Could you check a few things on this model? Use its own coordinates, in mm. A direction names the side the tool comes from. Coordinates: 2 decimals unless noted, no trailing zeros. Order: outer loops, then holes, each group sorted by start corner. A loop starts at its lowest first (then second) coordinate and runs counter-clockwise, first axis right, second up. Notation, with made-up numbers: (-2, -21) - (3, -21) arc R19 ccw to (3, -2) - close; hole circle Ø2 at (57, 7). An arc over 180 degrees is marked (long way). Answer as CSV lines item,"result". Start each with the question number.
1. I need wall thicknesses on probe 1 along X at (y, z) = (1.45, 24.65) (3 decimals); probe 2 along X at (y, z) = (28, 8.5) (3 decimals); probe 3 along Z at (x, y) = (-21, 22). Which ranges of each line are inside material? Lowest first, please.
2. I want a section at D-D, the plane z = -0.5. List the corners of the cut face in (x, y) for me (3 decimals).
3. Thinking about a two-plate mould opening in X: for faces 1 (the face through (38.82, 0.99, -26.08)), 2 (the face through (-49.775, 17, 0)), 3 (the face through (54, 2, -16)), 4 (the face through (39, 2, -24)), which applies, released by +X, released by -X, zero draft, split by the parting line, or undercut?
4. For pin 1 (5 mm diameter, centred on y = 18, z = -15.5, fed in from +X) (3 decimals); pin 2 (2 mm diameter, centred on y = 24.5, z = 2, fed in from -X) (3 decimals); pin 3 (1.3 mm diameter, centred on x = 40, z = -24.5, fed in from -Y), each with a flat end and sliding along its axis, tell me the tip position at first contact or that it passes through.
5. I want a section at C-C, the plane z = 24.65. List the corners of the cut face in (x, y) for me (3 decimals).
6. I want a section at A-A, the plane x = -42. List the corners of the cut face in (y, z) for me, and give its area (3 significant figures).
7. For faces 5 (the face through (50.775, 1, 0)), 6 (the face through (44.761, 0.986, 25.756)), 7 (the face through (53, 10, -16)), which set-ups out of +Z, -Z, +X, -X, +Y, -Y let a thin tool reach every point of the face, with its end or its side?
8. I want a section at B-B, the plane y = 18. List the corners of the cut face in (x, z) for me (3 decimals), and give its area (3 significant figures).
from build123d import *

# Parameters (mm, degrees)
ESBO_O1_W                  = 101.55
ESBO_O1_H                  = 53.3
RESSALTO_EXTRUS_O1_DEPTH   = 2
ESBO_O2_W                  = 53.2
ESBO_O2_H                  = 53.3
RESSALTO_EXTRUS_O2_DEPTH   = 26.416687688
CORTE_EXTRUS_O2_DEPTH      = 64.136079332
CORTE_EXTRUS_O2_DEPTH_BACK = 64.64
ESBO_O5_R                  = 1.5
ESBO_O6_W                  = 99.55
ESBO_O6_H                  = 51.3
RESSALTO_EXTRUS_O4_DEPTH   = 30
ESBO_O7_W                  = 16.925657076
ESBO_O7_H                  = 8.663776605
RESSALTO_EXTRUS_O5_DEPTH   = 8


with BuildPart() as part:
    # Esboço1 → Ressalto-extrusão1 (new body)
    with BuildSketch(Plane(origin=(0, 0, 0), x_dir=(1, 0, 0), z_dir=(0, 1, 0))):
        Rectangle(ESBO_O1_W, ESBO_O1_H)
    extrude(amount=RESSALTO_EXTRUS_O1_DEPTH)

    # Esboço2 → Ressalto-extrusão2 (add)
    with BuildSketch(Plane(origin=(0, 2, 0), x_dir=(1, 0, 0), z_dir=(0, 1, 0))):
        with Locations((6.175, 0)):
            Rectangle(ESBO_O2_W, ESBO_O2_H)
    extrude(amount=RESSALTO_EXTRUS_O2_DEPTH)

    # Esboço5 → Corte-extrusão2 (cut, two sides: drawn at the far end of the back side and taken through both)
    with BuildSketch(Plane(origin=(0, 2, 0), x_dir=(1, 0, 0), z_dir=(0, 1, 0)).offset(-CORTE_EXTRUS_O2_DEPTH_BACK)):
        with Locations(Location((-37.275, -24.65, 0), (0, 0, 90))):
            Circle(ESBO_O5_R)
        with Locations(Location((45.775, -24.65, 0), (0, 0, 90))):
            Circle(ESBO_O5_R)
        with Locations(Location((-36.275, 24.65, 0), (0, 0, 90))):
            Circle(ESBO_O5_R)
        with Locations(Location((39.275, 24.65, 0), (0, 0, 90))):
            Circle(ESBO_O5_R)
    extrude(amount=CORTE_EXTRUS_O2_DEPTH + CORTE_EXTRUS_O2_DEPTH_BACK, mode=Mode.SUBTRACT)

    # Esboço6 → Ressalto-extrusão4 (add)
    with BuildSketch(Plane(origin=(0, 2, 0), x_dir=(1, 0, 0), z_dir=(0, 1, 0))):
        Rectangle(ESBO_O6_W, ESBO_O6_H)
    extrude(amount=RESSALTO_EXTRUS_O4_DEPTH)

    # Esboço7 → Ressalto-extrusão5 (add)
    with BuildSketch(Plane(origin=(0, 2, 0), x_dir=(1, 0, 0), z_dir=(0, 1, 0))):
        with Locations((48.14371548, 15.499389289)):
            Rectangle(ESBO_O7_W, ESBO_O7_H)
    extrude(amount=RESSALTO_EXTRUS_O5_DEPTH)


solid = part.part
Solved:
1,probe 1,"x = -50.775 to -38.775, -35.775 to 44.275, 47.275 to 50.775"
1,probe 2,"x = -49.775 to 49.775"
1,probe 3,"z = -25.65 to 25.65"
2,outline,"(-50.775, 0) - (50.775, 0) - (50.775, 2) - (49.775, 2) - (49.775, 32) - (-49.775, 32) - (-49.775, 2) - (-50.775, 2) - close"
3,face 1,"undercut"
3,face 2,"released by -X"
3,face 3,"zero draft"
3,face 4,"undercut"
4,pin 1,"stops at x = 49.775"
4,pin 2,"stops at x = -49.775"
4,pin 3,"stops at y = 2"
5,outline,"(-50.775, 0) - (-38.775, 0) - (-38.775, 2) - (-35.775, 2) - (-35.775, 0) - (44.275, 0) - (44.275, 2) - (47.275, 2) - (47.275, 0) - (50.775, 0) - (50.775, 2) - (49.775, 2) - (49.775, 32) - (-49.775, 32) - (-49.775, 2) - (-50.775, 2) - close"
6,outline,"(0, -26.65) - (2, -26.65) - (2, -25.65) - (32, -25.65) - (32, 25.65) - (2, 25.65) - (2, 26.65) - (0, 26.65) - close"
6,area,"1,650 mm2"
7,face 5,"+Z, -Z, +X, -Y"
7,face 6,"-Y"
7,face 7,"+Z, -Z, +X, +Y"
8,outline,"(-49.775, -25.65) - (-20.425, -25.65) - (-20.425, -26.65) - (32.775, -26.65) - (32.775, -25.65) - (49.775, -25.65) - (49.775, 25.65) - (32.775, 25.65) - (32.775, 26.65) - (-20.425, 26.65) - (-20.425, 25.65) - (-49.775, 25.65) - close"
8,area,"5,210 mm2"
